```python
from build123d import *

# Parameters (mm, degrees)
EXTRUDE_2_DEPTH      = 10
SKETCH_3_R           = 3.5
SKETCH_3_R_2         = 20
SKETCH_3_R_3         = 2
SKETCH_3_R_4         = 12.5
CUT_EXTRUDE_1_DEPTH  = 660.636515889
SKETCH_6_W           = 10
SKETCH_6_H           = 50
CUT_EXTRUDE_14_DEPTH = 5
SKETCH_7_W           = 45
SKETCH_7_H           = 5
SKETCH_7_W_2         = 50
CUT_EXTRUDE_17_DEPTH = 660.636515889
SKETCH_4_R           = 2
CUT_EXTRUDE_18_DEPTH = 10
SKETCH_8_W           = 10
SKETCH_8_H           = 55
EXTRUDE_3_DEPTH      = 10
SKETCH_9_R           = 3.5
SKETCH_9_R_2         = 20
CUT_EXTRUDE_19_DEPTH = 660.636515889
EXTRUDE_4_DEPTH      = 10
SKETCH_14_R          = 20
SKETCH_14_R_2        = 3
CUT_EXTRUDE_20_DEPTH = 660.636515889
SKETCH_15_R          = 2
CUT_EXTRUDE_22_DEPTH = 660.636515889
CUT_EXTRUDE_26_DEPTH = 660.636515889


with BuildPart() as part:
    # 스케치1 → 보스-돌출2 (new body)
    with BuildSketch(Plane(origin=(0, 0, 0), x_dir=(0, 0, -1), z_dir=(1, 0, 0))):
        with BuildLine():
            Line((-350, -25), (353.480885827, -25))
            ThreePointArc((353.480885827, -25), (359.679041929, -24.015332259), (365.266885594, -21.158286093))
            Line((365.266885594, -21.158286093), (609.458437468, 155.703306991))
            ThreePointArc((609.458437468, 155.703306991), (620.947494037, 196.239910069), (580.410890959, 207.728966637))
            Line((580.410890959, 207.728966637), (150, 30))
            Line((150, 30), (-350, 30))
            Line((-350, 30), (-350, -25))
        make_face()
    extrude(amount=EXTRUDE_2_DEPTH)

    # 스케치3 → 컷-돌출1 (cut, through all)
    with BuildSketch(Plane(origin=(10, 0, 0), x_dir=(0, 0, -1), z_dir=(1, 0, 0))):
        with Locations((613.415951219, 194.53901549)):
            Circle(SKETCH_3_R)
        with Locations((570.305997446, 165.46098451)):
            Circle(SKETCH_3_R)
        with Locations((591.860974332, 180)):
            Circle(SKETCH_3_R_2)
        with Locations((337, -12)):
            Circle(SKETCH_3_R_3)
        with Locations((313, 12)):
            Circle(SKETCH_3_R_3)
        with Locations((313, -12)):
            Circle(SKETCH_3_R_3)
        with Locations((337, 12)):
            Circle(SKETCH_3_R_3)
        with Locations((325, 0)):
            Circle(SKETCH_3_R_4)
        with Locations((-313, -12)):
            Circle(SKETCH_3_R_3)
        with Locations((-313, 12)):
            Circle(SKETCH_3_R_3)
        with Locations((-325, 0)):
            Circle(SKETCH_3_R_4)
        with Locations((-337, -12)):
            Circle(SKETCH_3_R_3)
        with Locations((-337, 12)):
            Circle(SKETCH_3_R_3)
    extrude(amount=-CUT_EXTRUDE_1_DEPTH, mode=Mode.SUBTRACT)

    # 스케치6 → 컷-돌출14 (cut)
    with BuildSketch(Plane(origin=(0, 30, 0), x_dir=(1, 0, 0), z_dir=(0, 1, 0))):
        with Locations((5, -75)):
            Rectangle(SKETCH_6_W, SKETCH_6_H)
        with Locations((5, -275)):
            Rectangle(SKETCH_6_W, SKETCH_6_H)
        with Locations((5, 75)):
            Rectangle(SKETCH_6_W, SKETCH_6_H)
        with Locations((5, -175)):
            Rectangle(SKETCH_6_W, SKETCH_6_H)
    extrude(amount=-CUT_EXTRUDE_14_DEPTH, mode=Mode.SUBTRACT)

    # 스케치7 → 컷-돌출17 (cut, through all)
    with BuildSketch(Plane(origin=(10, 0, 0), x_dir=(0, 0, -1), z_dir=(1, 0, 0))):
        with Locations((177.5, 27.5)):
            Rectangle(SKETCH_7_W, SKETCH_7_H)
        with Locations((275, 27.5)):
            Rectangle(SKETCH_7_W_2, SKETCH_7_H)
    extrude(amount=-CUT_EXTRUDE_17_DEPTH, mode=Mode.SUBTRACT)

    # 스케치4 → 컷-돌출18 (cut)
    with BuildSketch(Plane(origin=(10, 0, 0), x_dir=(0, 0, -1), z_dir=(1, 0, 0))):
        with Locations((-237.5, 19)):
            Circle(SKETCH_4_R)
        with Locations(Location((-212.5, 19, 0), (0, 0, 180))):
            Circle(SKETCH_4_R)
        with Locations((-139.996213119, 19)):
            Circle(SKETCH_4_R)
        with Locations(Location((-114.996213119, 19, 0), (0, 0, 180))):
            Circle(SKETCH_4_R)
        with Locations((112.5, 19)):
            Circle(SKETCH_4_R)
        with Locations((212.5, 19)):
            Circle(SKETCH_4_R)
        with Locations(Location((237.5, 19, 0), (0, 0, 180))):
            Circle(SKETCH_4_R)
    extrude(amount=-CUT_EXTRUDE_18_DEPTH, mode=Mode.SUBTRACT)

    # 스케치8 → 보스-돌출3 (add)
    with BuildSketch(Plane.XY.offset(350)):
        with Locations((5, 2.5)):
            Rectangle(SKETCH_8_W, SKETCH_8_H)
    extrude(amount=EXTRUDE_3_DEPTH)

    # 스케치9 → 컷-돌출19 (cut, through all)
    with BuildSketch(Plane(origin=(10, 0, 0), x_dir=(0, 0, -1), z_dir=(1, 0, 0))):
        with Locations((-92.5, 0)):
            Circle(SKETCH_9_R)
        with Locations(Location((-40.5, 0, 0), (0, 0, 180))):
            Circle(SKETCH_9_R)
        with Locations(Location((-66.5, 0, 0), (0, 0, 180))):
            Circle(SKETCH_9_R_2)
        with Locations((155, 0)):
            Circle(SKETCH_9_R_2)
        with Locations((181, 0)):
            Circle(SKETCH_9_R)
        with Locations(Location((129, 0, 0), (0, 0, 180))):
            Circle(SKETCH_9_R)
    extrude(amount=-CUT_EXTRUDE_19_DEPTH, mode=Mode.SUBTRACT)

    # 스케치10 → 보스-돌출4 (add)
    with BuildSketch(Plane(origin=(0, 0, 0), x_dir=(0, 0, -1), z_dir=(1, 0, 0))):
        Polygon((100, 30), (100, 25), (50, 25), (50, 30), (-50, 30), (-360, 30), (-360, 100), (-50, 100), (319.520832407, 100), (150, 30), align=None)
    extrude(amount=EXTRUDE_4_DEPTH)

    # 스케치14 → 컷-돌출20 (cut, through all)
    with BuildSketch(Plane(origin=(10, 0, 0), x_dir=(0, 0, -1), z_dir=(1, 0, 0))):
        with Locations((44.25, 11)):
            Circle(SKETCH_14_R)
        with Locations((70.25, 11)):
            Circle(SKETCH_14_R_2)
        with Locations(Location((18.25, 11, 0), (0, 0, 180))):
            Circle(SKETCH_14_R_2)
    extrude(amount=-CUT_EXTRUDE_20_DEPTH, mode=Mode.SUBTRACT)

    # 스케치15 → 컷-돌출22 (cut, through all)
    with BuildSketch(Plane(origin=(10, 0, 0), x_dir=(0, 0, -1), z_dir=(1, 0, 0))):
        with Locations((331.433412373, 50.824001827)):
            Circle(SKETCH_15_R)
        with Locations((316.195018887, 87.807665301)):
            Circle(SKETCH_15_R)
        with Locations(Location((451.630318664, 100.348780655, 0), (0, 0, 180))):
            Circle(SKETCH_15_R)
        with Locations(Location((436.391925178, 137.332444129, 0), (0, 0, 180))):
            Circle(SKETCH_15_R)
    extrude(amount=-CUT_EXTRUDE_22_DEPTH, mode=Mode.SUBTRACT)

    # 스케치17 → 컷-돌출26 (cut, through all)
    with BuildSketch(Plane(origin=(10, 0, 0), x_dir=(0, 0, -1), z_dir=(1, 0, 0))):
        Polygon((134, 100), (144, 100), (144, 85), (124, 85), (124, 70.009449614), (144, 70.009449614), (144, 54.646019177), (124, 54.646019177), (124, 39.485590498), (144, 39.485590498), (144, 23.660735911), (134, 23.660735911), (134, -25.259204994), (-374.726859986, -25.259204994), (-374.726859986, 260.6847899), (134, 260.6847899), align=None)
    extrude(amount=-CUT_EXTRUDE_26_DEPTH, mode=Mode.SUBTRACT)


solid = part.part
```
Geometry: final body of the model. Coordinates: model frame, mm. A direction names the side the tool comes from. Round coordinates to 2 decimals unless told otherwise and drop trailing zeros. Order: outer loops, then holes, each group sorted by start corner. A loop starts at its lowest first (then second) coordinate and runs counter-clockwise, first axis right, second up. Notation, with made-up numbers: (-36.75, 38) -> (17.25, 38) arc R23 ccw to (17.25, 74) -> close; hole circle Ø2 at (75, -26.5). An arc over 180 degrees is marked (long way). Use one line per item in the form item = value. Start each with the question number.
1. Cut plane B-B (x = 3). Count the separate pieces of the cut face and the enclosed holes in it, then the cut area to 3 significant figures.
2. Cut plane A-A (z = -325). Return the cut outline in (x, y).
3. Cut plane D-D (y = 116). Return the cut outline in (x, z), then the cut area to 3 significant figures.
4. Line query: probe 1 along Y at (x, z) = (3.5, -181); probe 2 along Z at (x, y) = (3.5, 197); probe 3 along Y at (x, z) = (1.75, -262). Output: solid intervals per line, ascending.
5. Reachability of faces 4 (the face through (5, 93, -144)), 5 (the face through (5, 78, -124)), 6 (the face through (5, 62, -144)), 7 (the face through (0, 69, -378)), 8 (the face through (5, 30, -275)) from +Z, -Z, +X, -X, +Y, -Y: full face, straight path, thin tool, end or side. Return the list, or none.
6. Cut plane C-C (z = -477.5). Return the cut outline in (x, y).
7. Draft query along Z for faces 1 (the face through (5, 25, -275)), 2 (the face through (5, 47, -124)), 3 (the face through (5, 85, -134)). Return one class per face: pulls with the +Z half, pulls with the -Z half, needs draft (parallel to the pull), parting line crosses it, or undercut.
8. Pin query (flat end, axial travel): pin 1 Ø4 at (x, z) = (1, -366) entering from +Y; pin 2 Ø5 at (x, y) = (1.5, 106) entering from -Z; pin 3 Ø3.5 at (y, z) = (19, -212.5) entering from -X; pin 4 Ø5 at (x, z) = (3, -280.5) entering from +Y. Return the tip coordinate at first contact, or that it passes through.
Solution:
q1.separate_pieces = 1
q1.enclosed_holes = 18
q1.area = 50,800 mm^2
q2.outline = (0, -25) -> (10, -25) -> (10, -12.5) -> (0, -12.5) -> close; (0, 12.5) -> (10, 12.5) -> (10, 102.26) -> (0, 102.26) -> close
q3.outline = (0, -554.64) -> (10, -554.64) -> (10, -358.27) -> (0, -358.27) -> close
q3.area = 1,960 mm^2
q4.probe_1 = -25 to -3.5, 3.5 to 25, 30 to 100
q4.probe_2 = -620.51 to -615.9, -610.93 to -602.4, -581.33 to -554.43
q4.probe_3 = -25 to 25, 30 to 100
q5.face_4 = +Z, +X, -X, +Y
q5.face_5 = +Z, +X, -X, +Y, -Y
q5.face_6 = +Z, +X, -X
q5.face_7 = +Z, -Z, -X, +Y, -Y
q5.face_8 = +X, -X
q6.outline = (0, 60.13) -> (10, 60.13) -> (10, 165.23) -> (0, 165.23) -> close
q7.face_1 = undercut
q7.face_2 = pulls with the +Z half
q7.face_3 = needs draft
q8.pin_1 = 120.02
q8.pin_2 = -544.29
q8.pin_3 = through
q8.pin_4 = 100
